from build123d import *

# Parameters (mm, degrees)
F1_DEPTH      = 2
F2_R          = 1.4
F3_DEPTH      = 5
F5_DEPTH      = 1
F6_R          = 0.99999
F7_R          = 1
F8_R          = 2.25
F9_DEPTH      = 0.5
F10_S5_R      = 2.25
F10_T6_DEPTH  = 5
F10_S11_R     = 2.25
F10_T12_DEPTH = 5
F10_S17_R     = 2.25
F10_T18_DEPTH = 5
F10_S23_R     = 2.25
F10_T24_DEPTH = 5


# Not quite as in the source:
# - a fillet or chamfer that OpenCascade refuses, or shapes differently, is made with other operations: its cross-section is extruded or revolved along the edge and cut away or added
# - a fillet or chamfer is up to 0.001 mm smaller than in the source, because OpenCascade refuses the exact size


with BuildPart() as f1:
    # F0 (on Top) → F1 (new body)
    with BuildSketch(Plane.XY):
        with BuildLine():
            ThreePointArc((0, 3), (0.8786796564, 0.8786796564), (3, 0))
            Line((3, 0), (47, 0))
            ThreePointArc((47, 0), (49.1213203436, 0.8786796564), (50, 3))
            Line((50, 3), (50, 72))
            ThreePointArc((50, 72), (49.1213203436, 74.1213203436), (47, 75))
            Line((47, 75), (3, 75))
            ThreePointArc((3, 75), (0.8786796564, 74.1213203436), (0, 72))
            Line((0, 72), (0, 3))
        make_face()
    extrude(amount=F1_DEPTH)

    # F2 (on face) → F3 (cut)
    with BuildSketch(Plane.XY.offset(2)):
        with Locations((4, 71)):
            Circle(F2_R)
        with Locations((46, 71)):
            Circle(F2_R)
        with Locations((4, 4)):
            Circle(F2_R)
        with Locations((46, 4)):
            Circle(F2_R)
    extrude(amount=-F3_DEPTH, mode=Mode.SUBTRACT)

    # F4 (on face) → F5 (join)
    with BuildSketch(Plane.XY.offset(2)):
        with BuildLine():
            ThreePointArc((8, 5), (8.8786796564, 2.8786796564), (11, 2))
            Line((11, 2), (39, 2))
            ThreePointArc((39, 2), (41.1213203436, 2.8786796564), (42, 5))
            Line((42, 5), (42, 8))
            Line((42, 8), (45, 8))
            ThreePointArc((45, 8), (47.1213203436, 8.8786796564), (48, 11))
            Line((48, 11), (48, 64))
            ThreePointArc((48, 64), (47.1213203436, 66.1213203436), (45, 67))
            Line((45, 67), (42, 67))
            Line((42, 67), (42, 70))
            ThreePointArc((42, 70), (41.1213203436, 72.1213203436), (39, 73))
            Line((39, 73), (11, 73))
            ThreePointArc((11, 73), (8.8786796564, 72.1213203436), (8, 70))
            Line((8, 70), (8, 67))
            Line((8, 67), (5, 67))
            ThreePointArc((5, 67), (2.8786796564, 66.1213203436), (2, 64))
            Line((2, 64), (2, 11))
            ThreePointArc((2, 11), (2.8786796564, 8.8786796564), (5, 8))
            Line((5, 8), (8, 8))
            Line((8, 8), (8, 5))
        make_face()
    extrude(amount=F5_DEPTH)

    # F6 (radius 1 in the source; OpenCascade refuses exactly that, so slightly less here)
    f6_edges = [f1.edges().sort_by_distance(p)[0] for p in [
        (47.12132, 8.87868, 3),
        (43.5, 8, 3),
        (42, 6.5, 3),
        (41.12132, 2.87868, 3),
        (25, 2, 3),
        (8.87868, 2.87868, 3),
        (8, 6.5, 3),
        (6.5, 8, 3),
        (2.87868, 8.87868, 3),
        (2, 37.5, 3),
        (2.87868, 66.12132, 3),
        (6.5, 67, 3),
        (8, 68.5, 3),
        (8.87868, 72.12132, 3),
        (25, 73, 3),
        (41.12132, 72.12132, 3),
        (42, 68.5, 3),
        (43.5, 67, 3),
        (47.12132, 66.12132, 3),
        (48, 37.5, 3),
    ]]
    fillet(f6_edges, radius=F6_R)

    # F7
    f7_edges = [f1.edges().sort_by_distance(p)[0] for p in [
        (0, 37.5, 0),
    ]]
    fillet(f7_edges, radius=F7_R)

    # F8 (on face) → F9 (cut)
    with BuildSketch(Plane(origin=(0, 0, 0), x_dir=(1, 0, 0), z_dir=(0, 0, -1))):
        with Locations((4, -4)):
            Circle(F8_R)
        with Locations((46, -4)):
            Circle(F8_R)
        with Locations((46, -71)):
            Circle(F8_R)
        with Locations((4, -71)):
            Circle(F8_R)
    extrude(amount=-F9_DEPTH, mode=Mode.SUBTRACT)

    # F10: chamfer of 1 on 4 edges, made by hand


with BuildPart() as f10_tool2:
    # F10_s3 → F10_t4 (revolve)
    with BuildSketch(Plane.XZ.offset(-4)):
        Polygon((5.4, 1.5), (6.4, 0.5), (5.4, 0.5), align=None)
    revolve(axis=Axis((4, 4, 0.5), (0, 0, 1)))

    # F10_s5 → F10_t6 (intersect, symmetric)
    with BuildSketch(Plane.XY.offset(1)):
        with Locations((4, 4)):
            Circle(F10_S5_R)
    extrude(amount=F10_T6_DEPTH, both=True, mode=Mode.INTERSECT)


with BuildPart() as f1_1:
    add(f1.part)

    # F10_t1: cut F10_tool2
    add(f10_tool2.part, mode=Mode.SUBTRACT)


with BuildPart() as f10_tool8:
    # F10_s9 → F10_t10 (revolve)
    with BuildSketch(Plane.XZ.offset(-4)):
        Polygon((47.4, 1.5), (48.4, 0.5), (47.4, 0.5), align=None)
    revolve(axis=Axis((46, 4, 0.5), (0, 0, 1)))

    # F10_s11 → F10_t12 (intersect, symmetric)
    with BuildSketch(Plane.XY.offset(1)):
        with Locations((46, 4)):
            Circle(F10_S11_R)
    extrude(amount=F10_T12_DEPTH, both=True, mode=Mode.INTERSECT)


with BuildPart() as f1_2:
    add(f1_1.part)

    # F10_t7: cut F10_tool8
    add(f10_tool8.part, mode=Mode.SUBTRACT)


with BuildPart() as f10_tool14:
    # F10_s15 → F10_t16 (revolve)
    with BuildSketch(Plane.XZ.offset(-71)):
        Polygon((5.4, 1.5), (6.4, 0.5), (5.4, 0.5), align=None)
    revolve(axis=Axis((4, 71, 0.5), (0, 0, 1)))

    # F10_s17 → F10_t18 (intersect, symmetric)
    with BuildSketch(Plane.XY.offset(1)):
        with Locations((4, 71)):
            Circle(F10_S17_R)
    extrude(amount=F10_T18_DEPTH, both=True, mode=Mode.INTERSECT)


with BuildPart() as f1_3:
    add(f1_2.part)

    # F10_t13: cut F10_tool14
    add(f10_tool14.part, mode=Mode.SUBTRACT)


with BuildPart() as f10_tool20:
    # F10_s21 → F10_t22 (revolve)
    with BuildSketch(Plane.XZ.offset(-71)):
        Polygon((47.4, 1.5), (48.4, 0.5), (47.4, 0.5), align=None)
    revolve(axis=Axis((46, 71, 0.5), (0, 0, 1)))

    # F10_s23 → F10_t24 (intersect, symmetric)
    with BuildSketch(Plane.XY.offset(1)):
        with Locations((46, 71)):
            Circle(F10_S23_R)
    extrude(amount=F10_T24_DEPTH, both=True, mode=Mode.INTERSECT)


with BuildPart() as f1_4:
    add(f1_3.part)

    # F10_t19: cut F10_tool20
    add(f10_tool20.part, mode=Mode.SUBTRACT)


solid = f1_4.part
Check sheet for the modelled part. Datum: model origin and axes. Units: mm. A direction names the side the tool comes from. Give positions to 0.01 mm unless a question says otherwise; leave off trailing zeros. Answer as a JSON object with one key per item and string values. Group by question number.
Q1. Release check for a two-part mould opening along X. For faces 3 (the cylindrical face through (49.14, 74.1, 1.49)), 4 (the flat face through (1, 40, 2)), 5 (the cylindrical face through (46.65, 69.76, 1.75)) record: released by +X, released by -X, zero draft, split by the parting line, or undercut.
Q2. Go/stop test with a flat-tipped pin: P1, Ø3, axis at x = 46, y = 71, coming from the +Z side. Record where the tip stops, or that it passes through.
Q3. Cross-section at C-C on x = 46. Give the number of separate pieces and of enclosed holes in the cut face, then the cut area to 3 significant figures.
Q4. Access from +Z, -Z, +X, -X, +Y, -Y to the whole of each face (thin tool, end or side, straight path). Record for faces 1 (the cylindrical face through (45.512, 73.196, 0.32)), 2 (the cylindrical face through (49.1, 0.86, 1.49)).
Q5. Material ranges on line 1 along X through (y, z) = (71, 1.8); line 2 along Y through (x, z) = (46, 1.85); line 3 along X through (y, z) = (71, 0.5), recorded low to high. Write a range as [from, to].
Evaluation:
{
 "1": {"face 3": "released by +X", "face 4": "zero draft", "face 5": "undercut"},
 "2": {"P1": "stops at z = 2"},
 "3": {"separate pieces": "3", "enclosed holes": "0", "area": "193 mm2"},
 "4": {"face 1": "-Z", "face 2": "+Z, -Z, +X, -Y"},
 "5": {"line 1": "x = [0, 2.6], [5.4, 44.6], [47.4, 50]", "line 2": "y = [0, 2.6], [5.4, 69.6], [72.4, 75]", "line 3": "x = [0.13, 1.75], [6.25, 43.75], [48.25, 49.87]"}
}
